Build history of the part. All positions in model axes, mm. A direction names the side the tool comes from. Round coordinates to 2 decimals unless told otherwise and drop trailing zeros. Loops run counter-clockwise (first coordinate to the right, second up) from the corner with the lowest first, then second, coordinate; pieces in that order, holes last. Notation, with made-up numbers: (-28, 8.25) - (-6, 8.25) arc R12 cw to (-6, 16.25) - close; hole circle Ø9 at (-39.75, 15.25). An arc over 180 degrees is marked (long way). Use one line per item in the form item = value. Start each with the question number.
Q1. 3-axis set-ups, long thin cutter, end or side, ignore diameter. For faces 1 (the face through (0, -15, 89)), 2 (the face through (27.5, -2, 89)): which of +Z, -Z, +X, -X, +Y, -Y reach the whole face in a straight line?
Q2. Pin check, flat tips, straight feed: pin 1 (12 mm diameter, centred on x = -9.5, y = -13, fed in from +Z); pin 2 (10 mm diameter, centred on x = 11.5, z = 63.5, fed in from +Y). Stop position of each tip, or through.
Q3. Saw through at B-B (z = 84.5). Give the cut face in (x, y).
Q4. Saw through at C-C (x = -5.5). Give the cut face in (y, z), then the cut area to 3 significant figures.
Q5. Drill centre lines: line 1 (X direction, y = -9.5, z = 114); line 2 (Y direction, x = -16.5, z = 49). Where is each one in solid material? Low to high.
Q6. Saw through at A-A (y = -3). Give the cut face in (x, z).
Autodesk Inventor part; units mm, degrees
ref_plane "YZ Plane" through (0, 0, 0) normal (1, 0, 0) x (0, 1, 0)
ref_plane "XZ Plane" through (0, 0, 0) normal (0, 1, 0) x (-1, 0, 0)
ref_plane "XY Plane" through (0, 0, 0) normal (0, 0, 1) x (1, 0, 0)
sketch "Sketch1" plane through (0, 0, 0) normal (0, 0, 1) x (1, 0, 0)
  line L0 (22.5, 15) -> (-22.5, 15) construction
  line L1 (-22.5, 15) -> (-22.5, -15)
  line L2 (-22.5, -15) -> (22.5, -15)
  line L3 (22.5, -15) -> (22.5, 15)
  line L4 (22.5, 15) -> (-22.5, -15) construction
  line L5 (-22.5, 15) -> (22.5, -15) construction
  line L6 (-27.5, -20) -> (-27.5, 15)
  line L7 (-27.5, 20) -> (27.5, 20) construction
  line L8 (27.5, 20) -> (27.5, 15) construction
  line L9 (27.5, -20) -> (-27.5, -20)
  line L10 (-22.5, 15) -> (-27.5, 15)
  line L11 (22.5, 15) -> (27.5, 15)
  line L12 (-27.5, 15) -> (-27.5, 20) construction
  line L13 (27.5, 15) -> (27.5, -20)
  point P0 (0, 0)
  dimension "d0" = 45
  dimension "d1" = 30
  dimension "d2" = 5
  dimension "d3" = 5
  dimension "d4" = 5
  dimension "d5" = 40
extrude "Extrusion1" add sketch "Sketch1" along normal blind 180
properties part number "track z2053"
Report:
q1.face_1 = +Z, -Z, +Y
q1.face_2 = +Z, -Z, +X, +Y, -Y
q2.pin_1 = 180
q2.pin_2 = -15
q3.outline = (-27.5, -20) - (27.5, -20) - (27.5, 15) - (22.5, 15) - (22.5, -15) - (-22.5, -15) - (-22.5, 15) - (-27.5, 15) - close
q4.outline = (-20, 0) - (-15, 0) - (-15, 180) - (-20, 180) - close
q4.area = 900 mm²
q5.line_1 = -27.5 to -22.5, 22.5 to 27.5
q5.line_2 = -20 to -15
q6.outline = (-27.5, 0) - (-22.5, 0) - (-22.5, 180) - (-27.5, 180) - close; (22.5, 0) - (27.5, 0) - (27.5, 180) - (22.5, 180) - close
